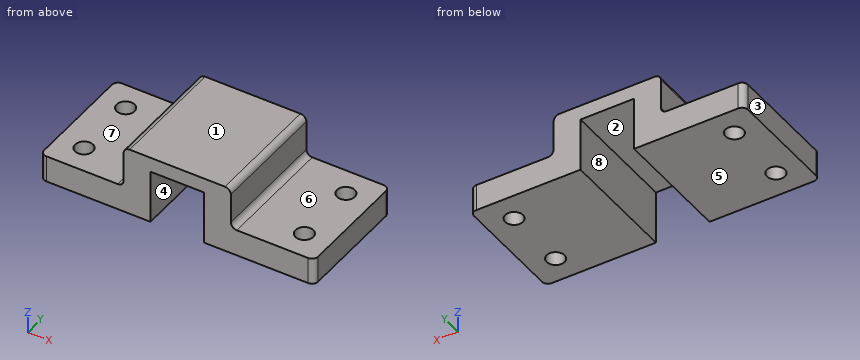
```python
from build123d import *

# Parameters (mm, degrees)
F1_DEPTH = 1016
F2_R     = 50.8
F3_R     = 50.8
F4_R     = 76.2
F5_DEPTH = 2286


with BuildPart() as f1:
    # F0 (on Front) → F1 (new body)
    with BuildSketch(Plane.XZ):
        Polygon((-939.8, 0), (0, 0), (0, 228.6), (-711.2, 228.6), (-711.2, 584.2), (-1625.6, 584.2), (-1625.6, 228.6), (-2336.8, 228.6), (-2336.8, 0), (-1397, 0), (-1397, 228.6), (-1397, 457.2), (-939.8, 457.2), (-939.8, 228.6), align=None)
    extrude(amount=F1_DEPTH)

    # F2
    f2_edges = [f1.edges().sort_by_distance(p)[0] for p in [
        (0, -1016, 114.3),
    ]]
    fillet(f2_edges, radius=F2_R)

    # F3
    f3_edges = [f1.edges().sort_by_distance(p)[0] for p in [
        (0, 0, 114.3),
        (-711.2, -508, 228.6),
        (-711.2, -508, 584.2),
        (-1625.6, -508, 584.2),
        (-1625.6, -508, 228.6),
        (-2336.8, 0, 114.3),
        (-2336.8, -1016, 114.3),
    ]]
    fillet(f3_edges, radius=F3_R)

    # F4 (on face) → F5 (cut)
    with BuildSketch(Plane.XY.offset(228.6)):
        with Locations((-228.6, -228.6)):
            Circle(F4_R)
        with Locations((-228.6, -787.4)):
            Circle(F4_R)
        with Locations((-2108.2, -787.4)):
            Circle(F4_R)
        with Locations((-2108.2, -228.6)):
            Circle(F4_R)
    extrude(amount=-F5_DEPTH, mode=Mode.SUBTRACT)


solid = f1.part
```
The listing builds one solid part. Answer for the finished solid, in the listing's coordinates (mm). Face numbers are marked on the shaded views. A direction names the side the tool comes from. Round coordinates to 2 decimals unless told otherwise and drop trailing zeros. Loops run counter-clockwise (first coordinate to the right, second up) from the corner with the lowest first, then second, coordinate; pieces in that order, holes last.
Q1. Section C-C, the plane z = 355.5 is taken. Determine the outline of the cut face in (x, y), then the cut area to 3 significant figures.
Q2. Which of the six approach directions +Z, -Z, +X, -X, +Y, -Y give full straight-line access (tool end or side, diameter ignored) to the marked faces 5, 6, 7 and 8?
Q3. Section B-B, the plane y = -228.6 is taken. Determine the outline of the cut face in (x, z).
Q4. Find the intervals of material crossed by line 1 (Y direction, x = -2108.2, z = 116); line 2 (X direction, y = -228, z = 76); line 3 (X direction, y = -120, z = 277), in increasing order.
Q5. For a pull along X with two mould halves and no side action, classify the marked faces 1, 2, 3 and 4 as released by +X, released by -X, zero draft, split by the parting line, or undercut.
Q6. Section A-A, the plane x = -228.6 is taken. Determine the outline of the cut face in (y, z).
Q7. Given pin 1 Ø8 at (x, y) = (-686, -189.5) entering from +Z; pin 2 Ø1.5 at (y, z) = (-134, 285.5) entering from -X; pin 3 Ø6 at (x, y) = (-367, -595.5) entering from +Z, each flat-ended and moving along its own axis, determine where each tip first touches the part or whether it passes through.
Q8. Section D-D, the plane y = -78.5 is taken. Determine the outline of the cut face in (x, z).
Completed:
1. outline: (-1625.6, -1016) - (-1397, -1016) - (-1397, 0) - (-1625.6, 0) - close; (-939.8, -1016) - (-711.2, -1016) - (-711.2, 0) - (-939.8, 0) - close
1. area: 465,000 mm2
2. face 5: -Z, +X, -X, +Y, -Y
2. face 6: +Z, +X, +Y, -Y
2. face 7: +Z, -X, +Y, -Y
2. face 8: -Z, +Y, -Y
3. outline: (-2336.8, 0) - (-2184.4, 0) - (-2184.4, 228.6) - (-2336.8, 228.6) - close; (-2032, 0) - (-1397, 0) - (-1397, 457.2) - (-939.8, 457.2) - (-939.8, 0) - (-304.8, 0) - (-304.8, 228.6) - (-660.4, 228.6) arc R50.8 cw to (-711.2, 279.4) - (-711.2, 533.4) arc R50.8 ccw to (-762, 584.2) - (-1574.8, 584.2) arc R50.8 ccw to (-1625.6, 533.4) - (-1625.6, 279.4) arc R50.8 cw to (-1676.4, 228.6) - (-2032, 228.6) - close; (-152.4, 0) - (0, 0) - (0, 228.6) - (-152.4, 228.6) - close
4. line 1: y = -1016 to -863.6, -711.2 to -304.8, -152.4 to 0
4. line 2: x = -2336.8 to -2184.4, -2032 to -1397, -939.8 to -304.8, -152.4 to 0
4. line 3: x = -1625.66 to -1397, -939.8 to -711.14
5. face 1: zero draft
5. face 2: undercut
5. face 3: released by -X
5. face 4: undercut
6. outline: (-1016, 0) - (-863.6, 0) - (-863.6, 228.6) - (-1016, 228.6) - close; (-711.2, 0) - (-304.8, 0) - (-304.8, 228.6) - (-711.2, 228.6) - close; (-152.4, 0) - (0, 0) - (0, 228.6) - (-152.4, 228.6) - close
7. pin 1: stops at z = 238.11
7. pin 2: stops at x = -1625.6
7. pin 3: stops at z = 228.6
8. outline: (-2336.8, 0) - (-1397, 0) - (-1397, 457.2) - (-939.8, 457.2) - (-939.8, 0) - (0, 0) - (0, 228.6) - (-660.4, 228.6) arc R50.8 cw to (-711.2, 279.4) - (-711.2, 533.4) arc R50.8 ccw to (-762, 584.2) - (-1574.8, 584.2) arc R50.8 ccw to (-1625.6, 533.4) - (-1625.6, 279.4) arc R50.8 cw to (-1676.4, 228.6) - (-2336.8, 228.6) - close
